Autodesk Inventor part; units mm, degrees
ref_plane "Work Plane1" through (100, 20, 0) normal (1, 0, 0) x (0, 0, -1)
ref_plane "YZ Plane" through (0, 0, 0) normal (1, 0, 0) x (0, 1, 0)
ref_plane "XZ Plane" through (0, 0, 0) normal (0, 1, 0) x (-1, 0, 0)
sketch "Sketch1" plane through (0, 0, 0) normal (0, 0, 1) x (1, 0, 0)
  line L0 (0, 0) -> (200, 0)
  line L1 (200, 0) -> (200, 370)
  line L2 (200, 370) -> (0, 370)
  line L3 (0, 370) -> (0, 0)
  circle A0 centre (17.5, 330) radius 7.6
  circle A1 centre (72.5, 330) radius 7.6
  circle A2 centre (127.5, 330) radius 7.6
  circle A3 centre (182.5, 330) radius 7.6
  circle A4 centre (45, 275) radius 7.6
  circle A5 centre (100, 275) radius 7.6
  circle A6 centre (155, 275) radius 7.6
  circle A7 centre (17.5, 220) radius 7.6
  circle A8 centre (72.5, 220) radius 7.6
  circle A9 centre (127.5, 220) radius 7.6
  circle A10 centre (182.5, 220) radius 7.6
  circle A11 centre (17.5, 110) radius 7.6
  circle A12 centre (72.5, 110) radius 7.6
  circle A13 centre (127.5, 110) radius 7.6
  circle A14 centre (182.5, 110) radius 7.6
  circle A15 centre (45, 165) radius 7.6
  circle A16 centre (100, 165) radius 7.6
  circle A17 centre (155, 165) radius 7.6
  line L4 (0, 370) -> (-2.5, 370)
  line L5 (-2.5, 370) -> (-2.5, 20)
  line L6 (-2.5, 20) -> (0, 20)
  line L7 (0, 20) -> (0, 370)
  line L8 (200, 370) -> (202.5, 370)
  line L9 (202.5, 370) -> (202.5, 20)
  line L10 (202.5, 20) -> (200, 20)
  line L11 (200, 20) -> (200, 370)
  point P0 (0, 20)
  dimension "d16" = 200
  dimension "d17" = 370
  dimension "d18" = 15.2
  dimension "d19" = 40
  dimension "d20" = 17.5
  dimension "d21" = 55
  dimension "d22" = 55
  dimension "d23" = 45
  dimension "d24" = 55
  dimension "d25" = 110
  dimension "d26" = 110
  dimension "d95" = 2.5
  dimension "d96" = 20
  dimension "d97" = 2.5
  dimension "d98" = 20
extrude "Plate1" add sketch "Sketch1" along normal blind 5 contours L3 L2 L1 L0 | L6 L5 L4 L3 | L1 L8 L9 L10 | A0 | A1 | A2 | A3
sketch "Sketch2" plane through (0, 0, 5) normal (0, 0, 1) x (1, 0, 0)
  line L0 (25, 47) -> (175, 47) construction
  line L1 (25, 39) -> (175, 39)
  line L2 (175, 55) -> (25, 55)
  arc A0 (25, 55) -> (25, 39) centre (25, 47) ccw
  arc A1 (175, 39) -> (175, 55) centre (175, 47) ccw
  line L3 (0, 0) -> (0, 20)
  line L4 (200, 20) -> (200, 0)
  circle A2 centre (127.5, 110) radius 7.6
  line L5 (200, 0) -> (0, 0)
  point P0 (100, 47)
  point P1 (0, 370)
  point P2 (200, 370)
  point P3 (100, 0)
  dimension "d32" = 16
  dimension "d35" = 55
  dimension "d39" = 150
extrude "Cut1" cut sketch "Sketch2" against normal through all contours A0 L2 A1 L1
sketch "Sketch3" plane through (0, 0, 5) normal (0, 0, 1) x (1, 0, 0)
  circle A0 centre (10, 40.1) radius 1.65
  line L0 (175, 39) -> (25, 39)
  line L1 (100, 39) -> (100, 0)
  line L2 (200, 0) -> (0, 0)
  circle A1 centre (190, 40.1) radius 1.65
  dimension "d41" = 3.3
  dimension "d47" = 180
  dimension "d48" = 1.1
extrude "Cut2" cut sketch "Sketch3" against normal blind 5
sketch "Sketch4" plane through (0, 0, 5) normal (0, 0, 1) x (1, 0, 0)
  line L0 (60, 322.5) -> (140, 322.5)
  line L1 (140, 322.5) -> (140, 287.5)
  line L2 (140, 287.5) -> (60, 287.5)
  line L3 (60, 287.5) -> (60, 322.5)
  line L4 (60, 322.5) -> (140, 287.5) construction
  line L5 (140, 322.5) -> (60, 287.5) construction
  line L6 (63.5, 317.5) -> (136.5, 317.5)
  line L7 (136.5, 317.5) -> (136.5, 292.5)
  line L8 (136.5, 292.5) -> (63.5, 292.5)
  line L9 (63.5, 292.5) -> (63.5, 317.5)
  line L10 (63.5, 317.5) -> (136.5, 292.5) construction
  line L11 (136.5, 317.5) -> (63.5, 292.5) construction
  line L12 (-2.5, 370) -> (202.5, 370)
  circle A0 centre (100, 275) radius 7.6
  circle A1 centre (137.5, 320.5) radius 1.65
  line L13 (100, 317.5) -> (100, 292.5)
  line L14 (63.5, 305) -> (136.5, 305)
  circle A2 centre (62.5, 320.5) radius 1.65
  circle A3 centre (137.5, 289.5) radius 1.65
  circle A4 centre (62.5, 289.5) radius 1.65
  point P0 (0, 0)
  point P1 (100, 305)
  point P2 (100, 305)
  point P3 (100, 370)
  point P4 (5, 370)
  point P5 (195, 370)
  point P6 (100, 305)
  dimension "d50" = 30
  dimension "d51" = 35
  dimension "d52" = 80
  dimension "d53" = 73
  dimension "d54" = 25
  dimension "d55" = 3.3
  dimension "d101" = 31
  dimension "d102" = 75
extrude "Extrusion1" cut sketch "Sketch4" against normal blind 10 contours L6 L13 L14 L9 | L6 L7 L14 L13 | L14 L13 L8 L9 | L14 L7 L8 L13 | A1 | A2 | A3 | A4
sketch "Sketch8" plane through (0, 0, 5) normal (0, 0, 1) x (1, 0, 0)
  line L0 (202.5, 370) -> (-2.5, 370)
  line L1 (196.5, 370) -> (199.5, 370)
  line L2 (199.5, 370) -> (199.5, 345)
  line L3 (199.5, 345) -> (196.5, 345)
  line L4 (196.5, 345) -> (196.5, 370)
  line L5 (200, 20) -> (200, 0)
  line L6 (202.5, 370) -> (202.5, 20)
  point P0 (0, 0)
  point P1 (195, 370)
  point P2 (5, 370)
  point P3 (200, 365)
  dimension "d76" = 25
  dimension "d77" = 3
  dimension "d99" = 3
extrude "Cut6" cut sketch "Sketch8" against normal blind 5
sketch "Sketch9" plane through (0, 0, 5) normal (0, 0, 1) x (1, 0, 0)
  line L0 (196.5, 370) -> (199.5, 370)
  line L1 (3.5, 370) -> (0.5, 370)
  line L2 (0.5, 370) -> (0.5, 345)
  line L3 (0.5, 345) -> (3.5, 345)
  line L4 (3.5, 345) -> (3.5, 370)
  line L5 (0, 0) -> (0, 20)
  line L6 (-2.5, 20) -> (-2.5, 370)
  point P0 (5, 370)
  point P1 (0, 365)
  point P2 (5, 370)
  dimension "d81" = 25
  dimension "d82" = 3
  dimension "d100" = 3
extrude "Cut7" cut sketch "Sketch9" against normal blind 5
sketch "Sketch10" plane through (0, 0, 5) normal (0, 0, 1) x (1, 0, 0)
  circle A0 centre (180, 10) radius 1.65
  line L0 (200, 20) -> (200, 0)
  line L1 (200, 0) -> (0, 0)
  circle A1 centre (20, 10) radius 1.65
  line L2 (0, 0) -> (0, 20)
  point P0 (200, 365)
  point P1 (0, 365)
  dimension "d86" = 3.3
  dimension "d88" = 10
  dimension "d89" = 3.3
  dimension "d90" = 10
  dimension "d91" = 20
  dimension "d94" = 20
extrude "Cut8" cut sketch "Sketch10" against normal blind 5
ref_plane "Work Plane1" through (100, 20, 0) normal (1, 0, 0) x (0, 0, -1)
equation "\"d97\" = d95"
equation "\"d98\" = d96"
equation "\"d36\" = Thickness"
equation "\"d45\" = Thickness"
equation "\"d79\" = Thickness"
equation "\"d84\" = Thickness"
equation "\"d92\" = Thickness"
equation "\"d31\" = Thickness"
equation "\"BendRadius\" = Thickness"
equation "\"BendReliefWidth\" = Thickness"
equation "\"BendReliefDepth\" = 0.5 * Thickness"
equation "\"TransitionRadius\" = BendRadius"
equation "\"JacobiRadiusSize\" = BendRadius"
equation "\"GapSize\" = Thickness"
properties part number "Random Plate  ( Laser Cut )"
Here's how the part is built. I have some questions about the finished solid (model axes, mm). A direction names the side the tool comes from. Coordinates: 2 decimals unless noted, no trailing zeros. Order: outer loops, then holes, each group sorted by start corner. A loop starts at its lowest first (then second) coordinate and runs counter-clockwise, first axis right, second up.
1) Which directions (+Z, -Z, +X, -X, +Y, -Y) give clear straight access to the entire face, cutting with the end or side of a thin tool? Please do faces 4 (the face through (99, 188, 0)), 5 (the face through (183, 47, 3)).
2) Imagine slicing it at C-C on z = 1.3. State how many separate pieces and enclosed holes the cut face has, and give its area (3 significant figures).
3) Imagine slicing it at A-A on y = 275. List the corners of the cut face in (x, z) for me.
4) I need wall thicknesses on line 1 (X direction, y = 320.5, z = 3.45); line 2 (X direction, y = 110.5, z = 4.5); line 3 (Y direction, x = 92, z = 0.45). Which ranges of each line are inside material? Lowest first, please.
5) We'd pull the mould along Y, two halves only. Please class faces 1 (the face through (99, 188, 5)), 2 (the face through (15.85, 227.42, 2.46)), 3 (the face through (16.511, 102.465, 2.465)): +Y half, -Y half, draft (parallel to the pull), parting line (faces both ways), or undercut.
6) Imagine slicing it at D-D on x = 71. List the corners of the cut face in (y, z) for me, and give its area (3 significant figures).
7) Will these pins go through, and if not, where does the flat tip stop? pin 1 (24.5 mm diameter, centred on x = 100, y = 165, fed in from +Z); pin 2 (1.5 mm diameter, centred on x = 2.5, z = 2.5, fed in from +Y); pin 3 (1.2 mm diameter, centred on x = -1, z = 3.5, fed in from -Y); pin 4 (2.5 mm diameter, centred on y = 5.5, z = 3, fed in from -X).
8) Imagine slicing it at B-B on x = 100. List the corners of the cut face in (y, z) for me.
Response values:
1. face 4: -Z, +X, -X, +Y, -Y
1. face 5: +Z, -Z
2. separate pieces: 1
2. enclosed holes: 24
2. area: 68,600 mm2
3. outline: (-2.5, 0) - (37.4, 0) - (37.4, 5) - (-2.5, 5) - close; (52.6, 0) - (92.4, 0) - (92.4, 5) - (52.6, 5) - close; (107.6, 0) - (147.4, 0) - (147.4, 5) - (107.6, 5) - close; (162.6, 0) - (202.5, 0) - (202.5, 5) - (162.6, 5) - close
4. line 1: x = -2.5 to 60.85, 64.15 to 135.85, 139.15 to 202.5
4. line 2: x = -2.5 to 9.92, 25.08 to 64.92, 80.08 to 119.92, 135.08 to 174.92, 190.08 to 202.5
4. line 3: y = 0 to 39, 55 to 292.5, 317.5 to 370
5. face 1: draft
5. face 2: undercut
5. face 3: undercut
6. outline: (0, 0) - (39, 0) - (39, 5) - (0, 5) - close; (55, 0) - (102.55, 0) - (102.55, 5) - (55, 5) - close; (117.45, 0) - (212.55, 0) - (212.55, 5) - (117.45, 5) - close; (227.45, 0) - (292.5, 0) - (292.5, 5) - (227.45, 5) - close; (317.5, 0) - (370, 0) - (370, 5) - (317.5, 5) - close
6. area: 1,500 mm2
7. pin 1: stops at z = 5
7. pin 2: stops at y = 345
7. pin 3: stops at y = 20
7. pin 4: stops at x = 0
8. outline: (0, 0) - (39, 0) - (39, 5) - (0, 5) - close; (55, 0) - (157.4, 0) - (157.4, 5) - (55, 5) - close; (172.6, 0) - (267.4, 0) - (267.4, 5) - (172.6, 5) - close; (282.6, 0) - (292.5, 0) - (292.5, 5) - (282.6, 5) - close; (317.5, 0) - (370, 0) - (370, 5) - (317.5, 5) - close
